```python
from build123d import *

# Parameters (mm, degrees)
SKETCH2_W           = 13
SKETCH2_H           = 13
BOSS_EXTRUDE1_DEPTH = 17.5
FILLET1_R           = 3
SKETCH3_R           = 4.6
SKETCH3_R_2         = 7
CUT_EXTRUDE1_DEPTH  = 16


with BuildPart() as part:
    # Sketch1 → Revolve4 (revolve)
    with BuildSketch(Plane(origin=(0, 0, 0), x_dir=(1, 0, 0), z_dir=(0, 1, 0))):
        with BuildLine():
            Line((0, 17.5), (0, -17.5))
            add(Edge.make_bspline(
                [(0, -17.5), (52.5, -17.5), (52.5, 0), (52.5, 17.5), (0, 17.5)],
                knots=[1.570796327, 1.570796327, 1.570796327, 3.141592654, 3.141592654, 4.71238898, 4.71238898, 4.71238898], degree=2, weights=[1, 0.707106781, 1, 0.707106781, 1]))
        make_face()
    revolve(axis=Axis((0, 0, -17.5), (0, 0, 1)))

    # Sketch2 → Boss-Extrude1 (add, through all)
    with BuildSketch(Plane.XY):
        Rectangle(SKETCH2_W, SKETCH2_H)
    extrude(amount=BOSS_EXTRUDE1_DEPTH)

    # Fillet1
    fillet1_edges = [part.edges().sort_by_distance(p)[0] for p in [
        (6.5, -6.5, 17.364828947),
        (-6.5, 6.5, 17.364828947),
        (6.5, 6.5, 17.364828947),
        (-6.5, -6.5, 17.364828947),
    ]]
    fillet(fillet1_edges, radius=FILLET1_R)

    # Sketch3 → Cut-Extrude1 (cut)
    with BuildSketch(Plane.XY.offset(8)):
        with Locations((0, 14)):
            Circle(SKETCH3_R)
        with Locations((10.945640755, 8.728857226)):
            Circle(SKETCH3_R)
        with Locations((13.648990771, -3.115293075)):
            Circle(SKETCH3_R)
        with Locations((6.074372348, -12.613564151)):
            Circle(SKETCH3_R)
        with Locations((-6.074372348, -12.613564151)):
            Circle(SKETCH3_R)
        with Locations((-13.648990771, -3.115293075)):
            Circle(SKETCH3_R)
        with Locations((-10.945640755, 8.728857226)):
            Circle(SKETCH3_R)
        Circle(SKETCH3_R_2)
    extrude(amount=-CUT_EXTRUDE1_DEPTH, mode=Mode.SUBTRACT)


solid = part.part
```
Here's how the part is built. I have some questions about the finished solid (model axes, mm). Round coordinates to 2 decimals unless told otherwise and drop trailing zeros.
Q1. Will these pins go through, and if not, where does the flat tip stop? P1, Ø3, axis at x = 6.5, y = -13, coming from the -Z side; P2, Ø4.5, axis at x = 12.5, y = -2, coming from the -Z side; P3, Ø7.5, axis at x = 7.5, y = -12, coming from the +Z side.
Q2. Please list where these lines run through material, in increasing order: probe 1 along Y at (x, z) = (0, -1.25); probe 2 along Y at (x, z) = (-7.5, -4.5); probe 3 along X at (y, z) = (-3, -5).
Q3. If we section it at A-A on x = 0: Give the number of separate pieces and of enclosed holes in the cut face, plus the area to 3 significant figures.
Answer below:
1. P1: stops at z = -16.95
1. P2: stops at z = -17.15
1. P3: stops at z = 17.15
2. probe 1: y = -52.37 to -7, 7 to 9.4, 18.6 to 52.37
2. probe 2: y = -50.18 to -16.99, -8.24 to 5.68, 11.78 to 50.18
2. probe 3: x = -50.22 to -18.25, -9.05 to -6.32, 6.32 to 9.05, 18.25 to 50.22
3. separate pieces: 1
3. enclosed holes: 2
3. area: 2,520 mm2
